Verification items for the finished model (mm, model axes). Give positions to 0.01 mm unless a question says otherwise; leave off trailing zeros. Loops run counter-clockwise (first coordinate to the right, second up) from the corner with the lowest first, then second, coordinate; pieces in that order, holes last. Notation, with made-up numbers: (51, -26.75) - (93, -26.75) arc R28 ccw to (93, 4.25) - close; hole circle Ø5 at (-39, 3.5). An arc over 180 degrees is marked (long way). Use one line per item in the form item = value.
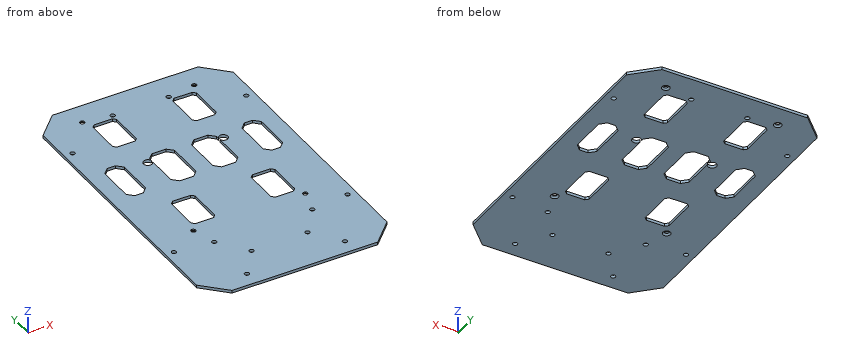
```python
from build123d import *

# Parameters (mm, degrees)
SKETCH_6_R               = 1.65
EXTRUDE_401_DEPTH        = 2
SKETCH_7_R               = 3.1
CUT_EXTRUDE_474_DEPTH    = 2
SKETCH_8_R               = 2.75
D5P5_1P1_DEPTH           = 1.1
D5P5_1P1_DRAFT           = 45
D5P5_1P1_PROFILE_2_DEPTH = 1.1
D5P5_1P1_PROFILE_2_DRAFT = 45
D5P5_1P1_PROFILE_3_DEPTH = 1.1
D5P5_1P1_PROFILE_3_DRAFT = 45
D5P5_1P1_PROFILE_4_DEPTH = 1.1
D5P5_1P1_PROFILE_4_DRAFT = 45


with BuildPart() as part:
    # 草图6 → Extrude 401 (new body)
    with BuildSketch(Plane.XY):
        Polygon((-52, -116), (52, -116), (68, -100), (68, 88), (52, 104), (-52, 104), (-68, 88), (-68, -100), align=None)
        with Locations((-20, -85)):
            Circle(SKETCH_6_R, mode=Mode.SUBTRACT)
        with Locations((-62, -62)):
            Circle(SKETCH_6_R, mode=Mode.SUBTRACT)
        with Locations((-40, -48)):
            Circle(SKETCH_6_R, mode=Mode.SUBTRACT)
        with Locations((-35, -105)):
            Circle(SKETCH_6_R, mode=Mode.SUBTRACT)
        with Locations((-20, 85)):
            Circle(SKETCH_6_R, mode=Mode.SUBTRACT)
        with Locations((-62, 62)):
            Circle(SKETCH_6_R, mode=Mode.SUBTRACT)
        with Locations((-40, 88)):
            Circle(SKETCH_6_R, mode=Mode.SUBTRACT)
        with Locations((-35, -65)):
            Circle(SKETCH_6_R, mode=Mode.SUBTRACT)
        with Locations((20, -85)):
            Circle(SKETCH_6_R, mode=Mode.SUBTRACT)
        with Locations((62, -62)):
            Circle(SKETCH_6_R, mode=Mode.SUBTRACT)
        with Locations((40, -48)):
            Circle(SKETCH_6_R, mode=Mode.SUBTRACT)
        with Locations((35, -105)):
            Circle(SKETCH_6_R, mode=Mode.SUBTRACT)
        with Locations((20, 85)):
            Circle(SKETCH_6_R, mode=Mode.SUBTRACT)
        with Locations((62, 62)):
            Circle(SKETCH_6_R, mode=Mode.SUBTRACT)
        with Locations((40, 88)):
            Circle(SKETCH_6_R, mode=Mode.SUBTRACT)
        with Locations((35, -65)):
            Circle(SKETCH_6_R, mode=Mode.SUBTRACT)
        Polygon((-35, -42), (-22, -42), (-20, -40), (-20, -16), (-22, -14), (-35, -14), (-37, -16), (-37, -40), align=None, mode=Mode.SUBTRACT)
        Polygon((-35, 54), (-22, 54), (-20, 56), (-20, 80), (-22, 82), (-35, 82), (-37, 80), (-37, 56), align=None, mode=Mode.SUBTRACT)
        Polygon((22, -42), (35, -42), (37, -40), (37, -16), (35, -14), (22, -14), (20, -16), (20, -40), align=None, mode=Mode.SUBTRACT)
        Polygon((22, 54), (35, 54), (37, 56), (37, 80), (35, 82), (22, 82), (20, 80), (20, 56), align=None, mode=Mode.SUBTRACT)
        Polygon((-20, 3), (-10, 3), (-6, 7), (-6, 33), (-10, 37), (-20, 37), (-24, 33), (-24, 7), align=None, mode=Mode.SUBTRACT)
        Polygon((-52, 3), (-46, 3), (-42, 7), (-42, 33), (-46, 37), (-52, 37), (-56, 33), (-56, 7), align=None, mode=Mode.SUBTRACT)
        Polygon((10, 3), (20, 3), (24, 7), (24, 33), (20, 37), (10, 37), (6, 33), (6, 7), align=None, mode=Mode.SUBTRACT)
        Polygon((46, 3), (52, 3), (56, 7), (56, 33), (52, 37), (46, 37), (42, 33), (42, 7), align=None, mode=Mode.SUBTRACT)
    extrude(amount=EXTRUDE_401_DEPTH)

    # 草图7 → Cut-Extrude 474 (cut)
    with BuildSketch(Plane.XY):
        with Locations((-27, -30)):
            Circle(SKETCH_7_R)
        with Locations((-27, 30)):
            Circle(SKETCH_7_R)
        with Locations((27, -30)):
            Circle(SKETCH_7_R)
        with Locations((27, 30)):
            Circle(SKETCH_7_R)
    extrude(amount=CUT_EXTRUDE_474_DEPTH, mode=Mode.SUBTRACT)


with BuildPart() as d5p5_1p1_tool:
    # 草图8 → 侧鞍下沉头孔_D5p5深1p1 (with draft: the straight prism first)
    with BuildSketch(Plane.XY):
        with Locations((-40, -48)):
            Circle(SKETCH_8_R)
    extrude(amount=D5P5_1P1_DEPTH)
    # 侧鞍下沉头孔_D5p5深1p1: the draft: its side faces are tilted about the plane it starts from
    d5p5_1p1_sides = [d5p5_1p1_tool.faces().sort_by_distance(p)[0] for p in [
        (-42.75, -48, 0.55),
    ]]
    draft(d5p5_1p1_sides, Plane.XY, D5P5_1P1_DRAFT)


with BuildPart() as part_1:
    add(part.part)

    # 侧鞍下沉头孔_D5p5深1p1: cut by d5p5_1p1_tool
    add(d5p5_1p1_tool.part, mode=Mode.SUBTRACT)


with BuildPart() as d5p5_1p1_profile_2_tool:
    # 草图8 → 侧鞍下沉头孔_D5p5深1p1 profile 2 (with draft: the straight prism first)
    with BuildSketch(Plane.XY):
        with Locations((-40, 88)):
            Circle(SKETCH_8_R)
    extrude(amount=D5P5_1P1_PROFILE_2_DEPTH)
    # 侧鞍下沉头孔_D5p5深1p1 profile 2: the draft: its side faces are tilted about the plane it starts from
    d5p5_1p1_profile_2_sides = [d5p5_1p1_profile_2_tool.faces().sort_by_distance(p)[0] for p in [
        (-42.75, 88, 0.55),
    ]]
    draft(d5p5_1p1_profile_2_sides, Plane.XY, D5P5_1P1_PROFILE_2_DRAFT)


with BuildPart() as part_2:
    add(part_1.part)

    # 侧鞍下沉头孔_D5p5深1p1 profile 2: cut by d5p5_1p1_profile_2_tool
    add(d5p5_1p1_profile_2_tool.part, mode=Mode.SUBTRACT)


with BuildPart() as d5p5_1p1_profile_3_tool:
    # 草图8 → 侧鞍下沉头孔_D5p5深1p1 profile 3 (with draft: the straight prism first)
    with BuildSketch(Plane.XY):
        with Locations((40, -48)):
            Circle(SKETCH_8_R)
    extrude(amount=D5P5_1P1_PROFILE_3_DEPTH)
    # 侧鞍下沉头孔_D5p5深1p1 profile 3: the draft: its side faces are tilted about the plane it starts from
    d5p5_1p1_profile_3_sides = [d5p5_1p1_profile_3_tool.faces().sort_by_distance(p)[0] for p in [
        (37.25, -48, 0.55),
    ]]
    draft(d5p5_1p1_profile_3_sides, Plane.XY, D5P5_1P1_PROFILE_3_DRAFT)


with BuildPart() as part_3:
    add(part_2.part)

    # 侧鞍下沉头孔_D5p5深1p1 profile 3: cut by d5p5_1p1_profile_3_tool
    add(d5p5_1p1_profile_3_tool.part, mode=Mode.SUBTRACT)


with BuildPart() as d5p5_1p1_profile_4_tool:
    # 草图8 → 侧鞍下沉头孔_D5p5深1p1 profile 4 (with draft: the straight prism first)
    with BuildSketch(Plane.XY):
        with Locations((40, 88)):
            Circle(SKETCH_8_R)
    extrude(amount=D5P5_1P1_PROFILE_4_DEPTH)
    # 侧鞍下沉头孔_D5p5深1p1 profile 4: the draft: its side faces are tilted about the plane it starts from
    d5p5_1p1_profile_4_sides = [d5p5_1p1_profile_4_tool.faces().sort_by_distance(p)[0] for p in [
        (37.25, 88, 0.55),
    ]]
    draft(d5p5_1p1_profile_4_sides, Plane.XY, D5P5_1P1_PROFILE_4_DRAFT)


with BuildPart() as part_4:
    add(part_3.part)

    # 侧鞍下沉头孔_D5p5深1p1 profile 4: cut by d5p5_1p1_profile_4_tool
    add(d5p5_1p1_profile_4_tool.part, mode=Mode.SUBTRACT)


solid = part_4.part
```
1. Section check D-D, the plane z = 0.8. State how many separate pieces and enclosed holes the cut face has, then the cut area to 3 significant figures.
Result set:
separate_pieces = 1
enclosed_holes = 24
area = 25,300 mm²
2. Section check C-C, the plane x = 48.5. Record the cut outline in (y, z).
Result set:
outline = (-116, 0) - (3, 0) - (3, 2) - (-116, 2) - close; (37, 0) - (104, 0) - (104, 2) - (37, 2) - close
3. Section check A-A, the plane x = 27. Record the cut outline in (y, z), then the cut area to 3 significant figures.
Result set:
outline = (-116, 0) - (-42, 0) - (-42, 2) - (-116, 2) - close; (-14, 0) - (26.9, 0) - (26.9, 2) - (-14, 2) - close; (33.1, 0) - (54, 0) - (54, 2) - (33.1, 2) - close; (82, 0) - (104, 0) - (104, 2) - (82, 2) - close
area = 316 mm²
4. Section check B-B, the plane y = -22. Record the cut outline in (x, z).
Result set:
outline = (-68, 0) - (-37, 0) - (-37, 2) - (-68, 2) - close; (-20, 0) - (20, 0) - (20, 2) - (-20, 2) - close; (37, 0) - (68, 0) - (68, 2) - (37, 2) - close
5. Scan lines: probe 1 along Y at (x, z) = (32, 1.45); probe 2 along Y at (x, z) = (35, 1.5); probe 3 along X at (y, z) = (16.5, 0.2). Record each from-to range of solid material in increasing order.
Result set:
probe_1 = -116 to -42, -14 to 54, 82 to 104
probe_2 = -116 to -106.65, -103.35 to -66.65, -63.35 to -42, -14 to 54, 82 to 104
probe_3 = -68 to -56, -42 to -24, -6 to 6, 24 to 42, 56 to 68
